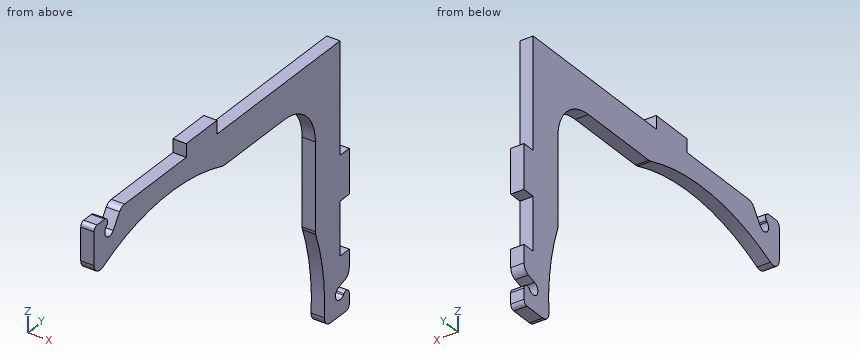
Autodesk Inventor part; units mm, degrees
ref_plane "YZ Plane" through (0, 0, 0) normal (1, 0, 0) x (0, 1, 0)
ref_plane "XZ Plane" through (0, 0, 0) normal (0, 1, 0) x (-1, 0, 0)
ref_plane "XY Plane" through (0, 0, 0) normal (0, 0, 1) x (1, 0, 0)
sketch "Sketch2" plane through (0, 0, 0) normal (1, 0, 0) x (0, 1, 0)
  line L0 (55, 30) -> (58, 30)
  line L1 (58, 30) -> (58, 20)
  line L2 (58, 20) -> (55, 20)
  line L3 (15, 55) -> (15, 58)
  line L4 (15, 58) -> (5, 58)
  line L5 (5, 58) -> (5, 55)
  line L6 (55, 30) -> (55, 55)
  line L7 (15, 55) -> (55, 55)
  line L8 (55, 20) -> (55, 8)
  line L9 (55, 8) -> (58, 8)
  arc A0 (54.5719, 1.4376) -> (56.0607, -1.0607) centre (55, 0) ccw
  line L10 (57, -5) -> (51.9134, -5)
  line L11 (56.5709, 2.033) -> (54.5719, 1.4376)
  line L12 (56.2929, -0.8284) -> (56.0607, -1.0607)
  line L13 (58, 8) -> (58, 3.9497)
  line L14 (58, -1.5355) -> (58, -4)
  arc A1 (56.5709, 2.033) -> (58, 3.9497) centre (56, 3.9497) ccw
  arc A2 (58, -1.5355) -> (56.2929, -0.8284) centre (57, -1.5355) ccw
  arc A3 (57, -5) -> (58, -4) centre (57, -4) ccw
  line L15 (-25, 54) -> (-25, 46.6369)
  arc A4 (-21.0607, 53.0607) -> (-18.7668, 51.146) centre (-20, 52) ccw
  line L16 (-20.8284, 53.2929) -> (-21.0607, 53.0607)
  line L17 (-16.6945, 54.1386) -> (-18.7668, 51.146)
  line L18 (5, 55) -> (-15.0503, 55)
  line L19 (-21.5355, 55) -> (-24, 55)
  arc A5 (-15.0503, 55) -> (-16.6945, 54.1386) centre (-15.0503, 53) ccw
  arc A6 (-25, 46.6369) -> (-22.1154, 44.8432) centre (-23, 46.6369) ccw
  arc A7 (-24, 55) -> (-25, 54) centre (-24, 54) ccw
  arc A8 (-20.8284, 53.2929) -> (-21.5355, 55) centre (-21.5355, 54) ccw
  arc A9 (49.9167, -2.8846) -> (47.1154, 16.7374) centre (0, 0) ccw
  arc A10 (16.7374, 47.1154) -> (-22.1154, 44.8432) centre (0, 0) ccw
  arc A11 (49.9167, -2.8846) -> (51.9134, -5) centre (51.9134, -3) ccw
  line L20 (47, 37) -> (47, 17.4069)
  line L21 (37, 47) -> (17.4069, 47)
  arc A12 (47, 17.4069) -> (47.1154, 16.7374) centre (49, 17.4069) ccw
  arc A13 (16.7374, 47.1154) -> (17.4069, 47) centre (17.4069, 49) ccw
  arc A14 (47, 37) -> (37, 47) centre (37, 37) ccw
  point P0 (-29.1247, 40.6418)
  point P1 (45.8258, -20)
  point P2 (49.96, -5)
  point P3 (-25, 43.3013)
  point P4 (58, -5)
  point P5 (-25, 55)
  point P6 (21.7945, 45)
  point P7 (45, 21.7945)
  point P8 (17.0587, 47)
  point P9 (47, 17.0587)
  point P10 (49.7494, -5)
  dimension "d5" = 10
  dimension "d6" = 10
  dimension "d13" = 40
  dimension "d14" = 25
  dimension "d15" = 3
  dimension "d16" = 3
  dimension "d22" = 55
  dimension "d23" = 55
  dimension "d43" = 12
  dimension "d44" = 3
  dimension "d46" = 3
  dimension "d48" = 3
  dimension "d53" = 2
  dimension "d54" = 1
  dimension "d57" = 80
  dimension "d58" = 3
  dimension "d59" = 5
  dimension "d61" = 3
  dimension "d64" = 2
  dimension "d65" = 2
  dimension "d66" = 1
  dimension "d67" = 3
  dimension "d75" = 4.0503
  dimension "d76" = 60
  dimension "d77" = 2
  dimension "d78" = 5
  dimension "d79" = 3
  dimension "d82" = 8
  dimension "d83" = 2
  dimension "d84" = 10
extrude "Extrusion3" add sketch "Sketch2" along normal blind 3
properties part number "OpenROV 2_2a Tube Brace"
Could you check a few things on this model? Use its own coordinates, in mm. Give positions to 0.01 mm unless a question says otherwise; leave off trailing zeros. Order: outer loops, then holes, each group sorted by start corner. A loop starts at its lowest first (then second) coordinate and runs counter-clockwise, first axis right, second up.
1. Will these pins go through, and if not, where does the flat tip stop? P1, Ø1.5, axis at x = 1, z = 12, coming from the +Y side; P2, Ø1.5, axis at x = 2, y = 43.5, coming from the +Z side; P3, Ø1.5, axis at x = 2, z = 31.5, coming from the -Y side.
2. I need wall thicknesses on L1, parallel to Y at x = 2.15, z = 34.5; L2, parallel to Y at x = 0.85, z = 53.5; L3, parallel to Y at x = 2.25, z = 52. Which ranges of each line are inside material? Lowest first, please.
3. Suppose I cut it at A-A (z = 52). List the corners of the cut face in (x, y) for me, plus the area to 3 significant figures.
4. Suppose I cut it at B-B (y = 18.5). List the corners of the cut face in (x, z) for me, plus the area to 3 significant figures.
Solved:
1. P1: stops at y = 55
1. P2: stops at z = 55
1. P3: stops at y = 47
2. L1: y = 47 to 55
2. L2: y = -25 to -20.67, -17.14 to 55
2. L3: y = -25 to -21.5, -18.18 to 55
3. outline: (0, -25) - (3, -25) - (3, -21.5) - (0, -21.5) - close; (0, -18.18) - (3, -18.18) - (3, 55) - (0, 55) - close
3. area: 230 mm2
4. outline: (0, 47) - (3, 47) - (3, 55) - (0, 55) - close
4. area: 24.0 mm2
